For this review, take the finished solid that the model builds, in its own axes (mm). A direction names the side the tool comes from. Coordinates: 2 decimals unless noted, no trailing zeros. Write each loop counter-clockwise with the first axis right and the second up, starting at its lowest first coordinate (ties: lowest second). Pieces come first, ordered by that corner, then holes. Notation, with made-up numbers: (14.25, 59.25) -> (19.25, 59.25) arc R6 ccw to (19.25, 67.25) -> close; hole circle Ø1 at (-20, 42.25). An arc over 180 degrees is marked (long way). One line per item, written item: value. Start each with the question number.
1) Add section D-D (x = 9). State the section outline as (y, z) points.
2) For probe 1 along X at (y, z) = (-2.5, 20); probe 2 along X at (y, z) = (1, 17.5); probe 3 along Z at (x, y) = (20.5, -5.25), list the stretches that pass through material, from the lowest coordinate up. Write a range as from..to.
3) Machinability: for faces 4 (the flat face through (18, -6, 10)), 5 (the cylindrical face through (57.717, 12.287, 23.202)), 6 (the flat face through (16, 3, 5)), which of the approach directions +Z, -Z, +X, -X, +Y, -Y give a long, thin tool a straight path to every point of the face, cutting with its end or side? Answer none if there is none.
4) For pin 1 Ø2 at (x, y) = (47.5, 2.5) entering from -Z; pin 2 Ø5 at (y, z) = (-7, 24.5) entering from +X; pin 3 Ø12 at (x, y) = (26.5, 10) entering from +Z, all flat-tipped, find the tip position at first contact; note any pin that passes through.
5) Add section B-B (y = -0.75). State how many separate pieces and enclosed holes the cut face has, and give its area (3 significant figures).
6) Add section A-A (x = 18). State the section outline as (y, z) points, and give its area (3 significant figures).
7) Mouldability with a two-part tool opening along X and no side actions: class faces 1 (the cylindrical face through (57.723, -12.287, 23.198)), 2 (the flat face through (37, 13, 14)), 3 (the cylindrical face through (32.608, 0.182, 10.652)) as released by +X, released by -X, zero draft, split by the parting line, or undercut.
8) Add section C-C (z = 34.5). State the section outline as (x, y) points, and give its area (3 significant figures).
from build123d import *

# Parameters (mm, degrees)
F1_DEPTH    = 13
F3_DEPTH    = 10.001
F4_R        = 5
F5_R        = 2.5
F6_T1_DEPTH = 42.5
F6_T4_ANGLE = 90
F6_T6_ANGLE = 90
F7_R        = 3.3
F8_DEPTH    = 58.201
F7_R_2      = 7.3
F10_DEPTH   = 4.4


# Not quite as in the source:
# - a fillet or chamfer that OpenCascade refuses, or shapes differently, is made with other operations: its cross-section is extruded or revolved along the edge and cut away or added


with BuildPart() as f1:
    # F0 (on Front) → F1 (new body, symmetric)
    with BuildSketch(Plane.XZ):
        Polygon((0, 10), (0, 0), (38.8, 0), (53.2, 24.941531629), (70.5205080757, 14.941531629), (75.5205080757, 23.6017856668), (49.5397459622, 38.6017856668), (33.0264973081, 10), align=None)
    extrude(amount=F1_DEPTH, both=True)

    # F2 (on face) → F3 (cut, through all)
    with BuildSketch(Plane.XY.offset(10)):
        with BuildLine():
            ThreePointArc((10, 3), (7, 0), (10, -3))
            Line((10, -3), (22, -3))
            ThreePointArc((22, -3), (25, 0), (22, 3))
            Line((22, 3), (10, 3))
        make_face()
    extrude(amount=-F3_DEPTH, mode=Mode.SUBTRACT)

    # F4
    f4_edges = [f1.edges().sort_by_distance(p)[0] for p in [
        (0, 0, 10),
        (33.026497, 0, 10),
    ]]
    fillet(f4_edges, radius=F4_R)

    # F5
    f5_edges = [f1.edges().sort_by_distance(p)[0] for p in [
        (0, 0, 0),
        (19.4, -13, 0),
        (19.4, 13, 0),
        (38.8, 0, 0),
        (46, -13, 12.470766),
        (46, 13, 12.470766),
        (53.2, 0, 24.941532),
        (61.860254, -13, 19.941532),
        (61.860254, 13, 19.941532),
        (70.520508, 0, 14.941532),
    ]]
    fillet(f5_edges, radius=F5_R)

    # F6: fillet of radius 13 on 2 edges, made by hand

    # F6_s2 → F6_t1 (cut)
    with BuildSketch(Plane(origin=(24.1, 0, 41.7424244624), x_dir=(0, 1, 0), z_dir=(0.5, 0, 0.8660254038))):
        with BuildLine():
            ThreePointArc((-13, -40.6017856668), (-9.1923881554, -49.7941738223), (0, -53.6017856668))
            Line((0, -53.6017856668), (-13, -53.6017856668))
            Line((-13, -53.6017856668), (-13, -40.6017856668))
        make_face()
        with BuildLine():
            ThreePointArc((13, -40.6017856668), (9.1923881554, -49.7941738223), (0, -53.6017856668))
            Line((0, -53.6017856668), (13, -53.6017856668))
            Line((13, -53.6017856668), (13, -40.6017856668))
        make_face()
    extrude(amount=F6_T1_DEPTH, mode=Mode.SUBTRACT)

    # F6_s3 → F6_t4 (revolve, cut)
    with BuildSketch(Plane(origin=(35.1621778265, 0, -20.3008928334), x_dir=(0, 1, 0), z_dir=(-0.8660254038, 0, 0.5))):
        with BuildLine():
            ThreePointArc((10.5, -48.2), (12.267766953, -48.932233047), (13, -50.7))
            Line((13, -50.7), (13, -48.2))
            Line((13, -48.2), (10.5, -48.2))
        make_face()
    revolve(axis=Axis((59.2621778265, 0, 21.441531629), (-0.5, 0, -0.8660254038)), revolution_arc=F6_T4_ANGLE, mode=Mode.SUBTRACT)

    # F6_s5 → F6_t6 (revolve, cut)
    with BuildSketch(Plane.XZ):
        with BuildLine():
            ThreePointArc((68.3554445662, 16.191531629), (70.252492179, 15.9417805727), (71.7705080757, 17.1065951385))
            Line((71.7705080757, 17.1065951385), (70.5205080757, 14.941531629))
            Line((70.5205080757, 14.941531629), (68.3554445662, 16.191531629))
        make_face()
    revolve(axis=Axis((59.2621778265, 0, 21.441531629), (-0.5, 0, -0.8660254038)), revolution_arc=F6_T6_ANGLE, mode=Mode.SUBTRACT)

    # F7 (on face) → F8 (cut, through all)
    with BuildSketch(Plane(origin=(29.1, 0, 50.4026785003), x_dir=(0.8660254038, 0, -0.5), z_dir=(0.5, 0, 0.8660254038))):
        with Locations((40.6017856668, 0)):
            Circle(F7_R)
    extrude(amount=-F8_DEPTH, mode=Mode.SUBTRACT)

    # F7 (on face) → F10 (cut)
    with BuildSketch(Plane(origin=(29.1, 0, 50.4026785003), x_dir=(0.8660254038, 0, -0.5), z_dir=(0.5, 0, 0.8660254038))):
        with Locations((40.6017856668, 0)):
            Circle(F7_R_2)
        with Locations((40.6017856668, 0)):
            Circle(F7_R, mode=Mode.SUBTRACT)
    extrude(amount=-F10_DEPTH, mode=Mode.SUBTRACT)


solid = f1.part
Numbers:
1. outline: (-13, 2.5) arc R2.5 ccw to (-10.5, 0) -> (-2.83, 0) -> (-2.83, 10) -> (-13, 10) -> close; (2.83, 0) -> (10.5, 0) arc R2.5 ccw to (13, 2.5) -> (13, 10) -> (2.83, 10) -> close
2. probe 1: 38.8..50.35, 61.76..73.16
2. probe 2: 37.36..48.9, 66.09..71.95
2. probe 3: 0..10
3. face 4: +Z, -X, +Y, -Y
3. face 5: -Z, +Y
3. face 6: +Z, -Z
4. pin 1: z = 13.34
4. pin 2: x = 74.81
4. pin 3: z = 10.59
5. separate pieces: 3
5. enclosed holes: 0
5. area: 634 mm²
6. outline: (-13, 2.5) arc R2.5 ccw to (-10.5, 0) -> (-3, 0) -> (-3, 10) -> (-13, 10) -> close; (3, 0) -> (10.5, 0) arc R2.5 ccw to (13, 2.5) -> (13, 10) -> (3, 10) -> close
6. area: 197 mm²
7. face 1: undercut
7. face 2: zero draft
7. face 3: released by -X
8. outline: (47.17, -13) -> (56.64, -13) -> (56.64, 13) -> (47.17, 13) -> close
8. area: 246 mm²
